Can you work these out from the model? Positions are in its coordinate system, mm. A direction names the side the tool comes from. Round coordinates to 2 decimals unless told otherwise and drop trailing zeros. Write each loop counter-clockwise with the first axis right and the second up, starting at its lowest first coordinate (ties: lowest second). Pieces come first, ordered by that corner, then holes. Notation, with made-up numbers: (48.25, 49.25) - (80.25, 49.25) arc R27 ccw to (80.25, 65.25) - close; hole circle Ø9 at (27, 55.25). An arc over 180 degrees is marked (long way). One line per item, written item: value. Start each with the question number.
(1) I want a section at B-B on x = -9. List the corners of the cut face in (y, z) for me.
(2) On a 3-axis mill with a long thin cutter (end or side, diameter ignored), from which of +Z, -Z, +X, -X, +Y, -Y can I reach the whole of each face in a straight line? I mean faces 1 (the face through (18, 0, 1)), 2 (the face through (49.004, -15.077, 1.521)), 3 (the face through (35.6, -30, 1)). Say none if no direction works.
(3) I want a section at C-C on y = 4.5. List the corners of the cut face in (x, z) for me.
(4) I want a section at A-A on x = 2.6. List the corners of the cut face in (y, z) for me, plus the area to 3 significant figures.
(5) I'm going to push flat-ended pins straight in: pin 1 Ø7.5 at (x, y) = (44.6, -13.25) entering from -Z; pin 2 Ø1.5 at (x, z) = (8, 1.5) entering from -Y. Where does each tip first touch, or does it pass through?
(6) If I drill on L1, parallel to X at y = -23, z = 2.25; L2, parallel to Y at x = 33.1, z = 1.3; L3, parallel to Y at x = -9, z = 0.9, over which ranges is the centre line in solid material (lowest first)? Write a range as from..to.
(7) I want a section at D-D on z = 1.1. Give the number of separate pieces and of enclosed holes in the cut face, plus the area to 3 significant figures.
Autodesk Inventor part; units mm, degrees
ref_plane "Work Plane1" through (0, 0, 0) normal (0, 0, 1) x (1, 0, 0)
ref_plane "Work Plane2" through (0, -26.08, 3) normal (0, 0, -1) x (0, 1, 0)
ref_plane "YZ Plane" through (0, 0, 0) normal (1, 0, 0) x (0, 1, 0)
ref_plane "Work Plane1" through (0, 0, 0) normal (0, 0, 1) x (1, 0, 0)
sketch "Sketch1" plane through (0, 0, 0) normal (0, 0, 1) x (1, 0, 0)
  line L0 (0, -26.08) -> (0, 0)
  line L1 (35.6, -26.08) -> (0, -26.08)
  line L2 (35.6, 0) -> (35.6, -26.08)
  line L3 (0, 0) -> (35.6, 0)
  point P0 (33.1, -3.1792)
  point P1 (33.1, -23.5192)
  point P2 (2.6, -23.48)
  point P3 (2.6, -3.14)
extrude "Extrusion1" add sketch "Sketch1" along normal blind 3
sketch "Sketch2" plane through (0, 0, 0) normal (0, 0, -1) x (-1, 0, 0)
  line L0 (-49.6, 16.67) -> (-39.6, 16.67)
  line L1 (-39.6, 16.67) -> (-35.6, 16.67)
  line L2 (-49.6, 16.67) -> (-53.6, 16.67)
  line L3 (-50.6, -33.042) -> (-53.6, -33.042)
  line L4 (-38.6, -33.042) -> (-35.6, -33.042)
  line L5 (4, 16.67) -> (0, 16.67)
  line L6 (4, 16.67) -> (14, 16.67)
  line L7 (14, 16.67) -> (18, 16.67)
  line L8 (15, -33.042) -> (18, -33.042)
  line L9 (3, -33.042) -> (0, -33.042)
  line L10 (0, 16.67) -> (0, -33.042)
  line L11 (-35.6, -33.042) -> (-35.6, 16.67)
  circle A0 centre (-44.6, 6.817) radius 1.45
  circle A1 centre (-44.6001, -23.183) radius 1.4501
  circle A2 centre (9, -23.183) radius 1.45
  circle A3 centre (9, 6.817) radius 1.45
  line L12 (-53.6, 16.67) -> (-53.6, -33.042)
  line L13 (-35.6, -26.08) -> (-35.6, 0)
  line L14 (-35.6, 0) -> (-35.6, -26.08)
  line L15 (-38.6, -33.042) -> (-50.6, -33.042)
  line L16 (3, -33.042) -> (15, -33.042)
  line L17 (18, -33.042) -> (18, 16.67)
  point P0 (0, 0)
ref_plane "Work Plane2" through (0, -26.08, 3) normal (0, 0, -1) x (0, 1, 0)
extrude "Extrusion2" add sketch "Sketch2" against normal up to surface (3 mm away)
sketch "Sketch3" plane through (0, 0, 3) normal (0, 0, 1) x (1, 0, 0)
  circle A0 centre (2.6, -22.94) radius 1.6
  circle A1 centre (33.1, -22.9008) radius 1.6
  circle A2 centre (33.1, -2.5608) radius 1.6
  circle A3 centre (2.6, -2.6) radius 1.6
  circle A4 centre (2.6, -2.6) radius 1.45
  circle A5 centre (2.6, -22.94) radius 1.45
  circle A6 centre (33.1, -22.9008) radius 1.45
  circle A7 centre (33.1, -2.5608) radius 1.45
  point P0 (0, 0)
  dimension "d8" = 2.9
  dimension "d9" = 2.9
  dimension "d10" = 2.9
  dimension "d11" = 2.9
extrude "Extrusion3" cut sketch "Sketch3" against normal through all contours A4 | A5 | A6 | A7
sketch "Sketch4" plane through (0, 0, 3) normal (0, 0, 1) x (1, 0, 0)
  circle A0 centre (-9, -23.183) radius 1.45
  line L0 (-9, -23.183) -> (-9, -13.251)
  circle A1 centre (-9, -13.251) radius 4.767
  circle A2 centre (44.6001, -23.183) radius 1.4501
  line L1 (44.6001, -23.183) -> (44.6001, -13.251)
  circle A3 centre (44.6001, -13.251) radius 4.767
  point P0 (0, 0)
  dimension "d14" = 9.932
  dimension "d15" = 9.534
  dimension "d16" = 9.534
extrude "Extrusion4" cut sketch "Sketch4" against normal through all contours A1 | A3
properties part number "gps_plate"
Established:
1. outline: (-33.04, 0) - (-24.63, 0) - (-24.63, 3) - (-33.04, 3) - close; (-21.73, 0) - (-18.02, 0) - (-18.02, 3) - (-21.73, 3) - close; (-8.48, 0) - (5.37, 0) - (5.37, 3) - (-8.48, 3) - close; (8.27, 0) - (16.67, 0) - (16.67, 3) - (8.27, 3) - close
2. face 1: +Z, -Z, +Y
2. face 2: +Z, -Z
2. face 3: +Z, -Z, -Y
3. outline: (-18, 0) - (0, 0) - (0, 3) - (-18, 3) - close; (35.6, 0) - (53.6, 0) - (53.6, 3) - (35.6, 3) - close
4. outline: (-26.08, 0) - (-24.39, 0) - (-24.39, 3) - (-26.08, 3) - close; (-21.49, 0) - (-4.05, 0) - (-4.05, 3) - (-21.49, 3) - close; (-1.15, 0) - (0, 0) - (0, 3) - (-1.15, 3) - close
4. area: 60.8 mm2
5. pin 1: through
5. pin 2: y = -26.08
6. L1: -18..-10.44, -7.56..1.15, 4.05..31.65, 34.55..43.16, 46.04..53.6
6. L2: -26.08..-24.35, -21.45..-4.01, -1.11..0
6. L3: -33.04..-24.63, -21.73..-18.02, -8.48..5.37, 8.27..16.67
7. separate pieces: 1
7. enclosed holes: 10
7. area: 2,520 mm2
